Design review of the part built by this model. Coordinates are the model's own, in mm. Face numbers are marked on the shaded views. Round coordinates to 2 decimals unless told otherwise and drop trailing zeros. Loops run counter-clockwise (first coordinate to the right, second up) from the corner with the lowest first, then second, coordinate; pieces in that order, holes last. Notation, with made-up numbers: (29.25, -37) - (38.25, -37) arc R28 ccw to (38.25, -14) - close; hole circle Ø2 at (22, 60). An arc over 180 degrees is marked (long way). Return JSON: item names as keys, results as strings. Group by question number.
(1) We need section B-B, the plane y = 0. Write out the cut boundary in (x, z).
(2) We need section C-C, the plane z = -4.75. Write out the cut boundary in (x, y) (1 decimal).
(3) Wall thickness on L1, parallel to Y at x = -39, z = -1.25; L2, parallel to X at y = -29.5, z = -1; L3, parallel to Y at x = -42, z = -1: over which ranges is each line inside the solid? List them lowest first. Write a range as [from, to].
(4) We need section A-A, the plane x = 0. Write out the cut boundary in (y, z).
(5) We need section D-D, the plane y = 13.5. Give the number of separate pieces and of enclosed holes in the cut face, and give its area (3 significant figures).
(6) The part is to be moulded in two halves that separate along Y. For the marked faces 1, 2 and 3, say which applies: pulls with the +Y half, pulls with the -Y half, needs draft (parallel to the pull), parting line crosses it, or undercut.
(7) Clearance check with flat-ended pins moving along their axes: pin 1 (1.5 mm diameter, centred on x = -44.5, y = 10.5, fed in from -Z); pin 2 (1 mm diameter, centred on y = 15.5, z = -3, fed in from -X); pin 3 (14.5 mm diameter, centred on x = -25, y = 16.5, fed in from -Z). State where each tip first meets the part, or that it passes through.
from build123d import *

# Parameters (mm, degrees)
SKETCH2_R          = 7.9375
CUT_EXTRUDE1_DEPTH = 85.463711951


with BuildPart() as part:
    # Sketch1 → Revolve1 (revolve)
    with BuildSketch(Plane(origin=(0, 0, 0), x_dir=(0, 0, -1), z_dir=(1, 0, 0)), mode=Mode.PRIVATE) as revolve1_sk:
        with BuildLine():
            Line((0, 0), (0, 52.809927725))
            ThreePointArc((0, 52.809927725), (0.130798304, 53.244522907), (0.479738309, 53.534733247))
            Line((0.479738309, 53.534733247), (0.872854821, 53.701601306))
            ThreePointArc((0.872854821, 53.701601306), (1.6002, 54.8005), (0.872854821, 55.899398694))
            Line((0.872854821, 55.899398694), (0.479738309, 56.066266753))
            ThreePointArc((0.479738309, 56.066266753), (0.130798304, 56.356477093), (0, 56.791072275))
            Line((0, 56.791072275), (0, 59.4614))
            Line((0, 59.4614), (2.8448, 59.4614))
            Line((2.8448, 59.4614), (7.9248, 45.504214709))
            Line((7.9248, 45.504214709), (7.9248, 0))
            Line((7.9248, 0), (0, 0))
        make_face()
    revolve(revolve1_sk.sketch.rotate(Axis((0, 0, 0), (0, 0, -1)), 90), axis=Axis((0, 0, 0), (0, 0, -1)))

    # Sketch2 → Cut-Extrude1 (cut, through all)
    with BuildSketch(Plane(origin=(0, 0, -7.9248), x_dir=(-1, 0, 0), z_dir=(0, 0, -1))):
        with Locations((-25, 16.5)):
            Circle(SKETCH2_R)
        with Locations((0, 30.6)):
            Circle(SKETCH2_R)
        with Locations((25, 16.5)):
            Circle(SKETCH2_R)
        Circle(SKETCH2_R)
    extrude(amount=-CUT_EXTRUDE1_DEPTH, mode=Mode.SUBTRACT)


solid = part.part
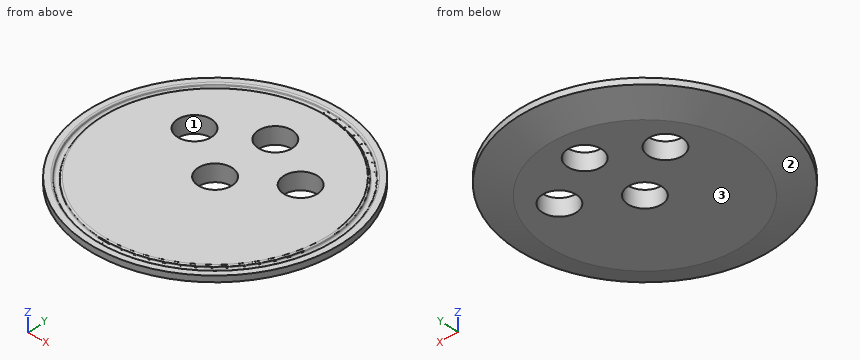
Solutions:
{
 "1": {"outline": "(-59.46, -2.84) - (-45.5, -7.92) - (-7.94, -7.92) - (-7.94, 0) - (-52.81, 0) arc R0.79 ccw to (-53.53, -0.48) - (-53.7, -0.87) arc R1.19 cw to (-55.9, -0.87) - (-56.07, -0.48) arc R0.79 ccw to (-56.79, 0) - (-59.46, 0) - close; (7.94, -7.92) - (45.5, -7.92) - (59.46, -2.84) - (59.46, 0) - (56.79, 0) arc R0.79 ccw to (56.07, -0.48) - (55.9, -0.87) arc R1.19 cw to (53.7, -0.87) - (53.53, -0.48) arc R0.79 ccw to (52.81, 0) - (7.94, 0) - close"},
 "2": {"outline": "circle Ø108.5 at (0, 0); hole circle Ø15.9 at (-25, 16.5); hole circle Ø15.9 at (0, 0); hole circle Ø15.9 at (0, 30.6); hole circle Ø15.9 at (25, 16.5)"},
 "3": {"L1": "[-44.88, -39.69], [-37.29, 37.29], [39.69, 44.88]", "L2": "[-51.63, -47.41], [-44.95, 44.95], [47.41, 51.63]", "L3": "[-42.09, -36.79], [-33.57, 33.57], [36.79, 42.09]"},
 "4": {"outline": "(-59.46, -2.84) - (-45.5, -7.92) - (-7.94, -7.92) - (-7.94, 0) - (-52.81, 0) arc R0.79 ccw to (-53.53, -0.48) - (-53.7, -0.87) arc R1.19 cw to (-55.9, -0.87) - (-56.07, -0.48) arc R0.79 ccw to (-56.79, 0) - (-59.46, 0) - close; (7.94, -7.92) - (22.66, -7.92) - (22.66, 0) - (7.94, 0) - close; (38.54, -7.92) - (45.5, -7.92) - (59.46, -2.84) - (59.46, 0) - (56.79, 0) arc R0.79 ccw to (56.07, -0.48) - (55.9, -0.87) arc R1.19 cw to (53.7, -0.87) - (53.53, -0.48) arc R0.79 ccw to (52.81, 0) - (38.54, 0) - close"},
 "5": {"separate pieces": "3", "enclosed holes": "0", "area": "604 mm^2"},
 "6": {"face 1": "undercut", "face 2": "parting line crosses it", "face 3": "needs draft"},
 "7": {"pin 1": "z = -7.92", "pin 2": "x = -57.53", "pin 3": "through"}
}
